Check sheet for the modelled part. Datum: model origin and axes. Units: mm. A direction names the side the tool comes from. Give positions to 0.01 mm unless a question says otherwise; leave off trailing zeros. Loops run counter-clockwise (first coordinate to the right, second up) from the corner with the lowest first, then second, coordinate; pieces in that order, holes last. Notation, with made-up numbers: M 89,-32 L 126,-32 A22 cw 126,-17 Z; hole C 58,26 d2. An arc over 180 degrees is marked long. Write each question's results on one line, items separated by ' | '. Start each with the question number.
1. Sectioned sample at C-C on x = 27. Record the cut outline in (y, z), and give its area (3 significant figures).
2. Material ranges on line 1 along Y through (x, z) = (-36, 9); line 2 along Z through (x, y) = (-46.5, 4.4), recorded low to high.
3. Sectioned sample at A-A on y = 4. Give the number of separate pieces and of enclosed holes in the cut face, and give its area (3 significant figures).
4. Sectioned sample at B-B on z = 18. Record the cut outline in (x, y), and give its area (3 significant figures).
5. Go/stop test with flat-tipped pins: pin 1 (2 mm diameter, centred on x = -43.5, y = -4, fed in from +Z); pin 2 (8 mm diameter, centred on x = -44.5, z = 7.5, fed in from -Y); pin 3 (5 mm diameter, centred on x = -46.5, z = 5, fed in from +Y). Record where each tip stops, or that it passes through.
6. Tool access check on faces 1 (the flat face through (-44, -6.2, 5)), 2 (the flat face through (-43, -4, 10)), 3 (the flat face through (-1, -38, 12)). Record the directions out of +Z, -Z, +X, -X, +Y, -Y that give a thin tool (end or side, any length) a straight path to the whole face; none if there is none.
7. Draft check along Y on faces 4 (the flat face through (-44, 6.2, 5)), 5 (the flat face through (-38, -1, 12)), 6 (the flat face through (-39, 3, 0)). Enter one of: pulls with the +Y half, pulls with the -Y half, needs draft (parallel to the pull), parting line crosses it, or undercut.
```python
from build123d import *

# Parameters (mm, degrees)
F0_W     = 80
F0_H     = 80
F0_W_2   = 76
F0_H_2   = 76
F1_DEPTH = 25
F2_W     = 12.4
F2_H     = 10
F3_DEPTH = 11.5
F4_R     = 4.99999
F5_R     = 1.9
F6_DEPTH = 25
F7_W     = 6.50001
F7_H     = 4.2
F7_W_2   = 4.99999
F8_DEPTH = 25


# Not quite as in the source:
# - a fillet or chamfer is up to 0.001 mm smaller than in the source, because OpenCascade refuses the exact size


with BuildPart() as f1:
    # F0 (on Top) → F1 (new body)
    with BuildSketch(Plane.XY):
        Rectangle(F0_W, F0_H)
        Rectangle(F0_W_2, F0_H_2, mode=Mode.SUBTRACT)
    extrude(amount=F1_DEPTH)

    # F2 (on face) → F3 (join)
    with BuildSketch(Plane(origin=(-40, 0, 0), x_dir=(0, -1, 0), z_dir=(-1, 0, 0))):
        with Locations((0, 5)):
            Rectangle(F2_W, F2_H)
    extrude(amount=F3_DEPTH)

    # F4 (radius 5 in the source; OpenCascade refuses exactly that, so slightly less here)
    f4_edges = [f1.edges().sort_by_distance(p)[0] for p in [
        (-51.5, 0, 10),
        (-51.5, 0, 0),
    ]]
    fillet(f4_edges, radius=F4_R)

    # F5 (on face) → F6 (cut)
    with BuildSketch(Plane(origin=(0, 6.2, 0), x_dir=(-1, 0, 0), z_dir=(0, 1, 0))):
        with Locations((46.5, 5)):
            Circle(F5_R)
    extrude(amount=-F6_DEPTH, mode=Mode.SUBTRACT)

    # F7 (on face) → F8 (cut)
    with BuildSketch(Plane.XY.offset(10)):
        with Locations((-43.250005, 0)):
            Rectangle(F7_W, F7_H)
        with Locations((-49.000005, 0)):
            Rectangle(F7_W_2, F7_H)
    extrude(amount=-F8_DEPTH, mode=Mode.SUBTRACT)


solid = f1.part
```
Output values:
1) outline: M -40,0 L -38,0 L -38,25 L -40,25 Z; M 38,0 L 40,0 L 40,25 L 38,25 Z | area: 100 mm2
2) line 1: -40 to -38, 38 to 40 | line 2: 0 to 3.1, 6.9 to 10
3) separate pieces: 2 | enclosed holes: 1 | area: 193 mm2
4) outline: M -40,-40 L 40,-40 L 40,40 L -40,40 Z; hole M -38,-38 L 38,-38 L 38,38 L -38,38 Z | area: 624 mm2
5) pin 1: z = 10 | pin 2: y = -6.2 | pin 3: y = 6.2
6) face 1: +Z, -Z, -X, -Y | face 2: +Z, -X, +Y, -Y | face 3: +Z, -Z
7) face 4: pulls with the +Y half | face 5: undercut | face 6: needs draft
